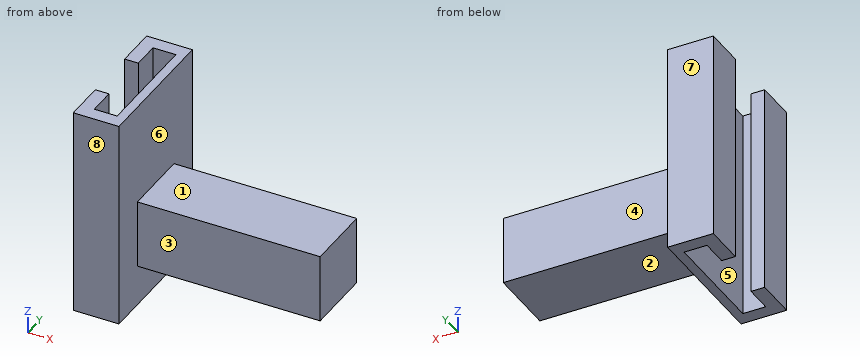
```python
from build123d import *

# Parameters (mm, degrees)
PAD_DEPTH    = 46
SKETCH002_W  = 14.95
SKETCH002_H  = 14.95
PAD001_DEPTH = 40


with BuildPart() as part:
    # Sketch → Pad (new body)
    with BuildSketch(Plane.XY):
        Polygon((-10, 15), (0, 15), (0, -15), (-10, -15), (-10, -6), (-7, -6), (-7, -12), (-2, -12), (-2, 12), (-7, 12), (-7, 6), (-10, 6), align=None)
    extrude(amount=PAD_DEPTH)

    # Sketch002 (on Face2 of Pad) → Pad001 (join)
    with BuildSketch(Plane.YZ):
        with Locations((0, 16.475)):
            Rectangle(SKETCH002_W, SKETCH002_H)
    extrude(amount=PAD001_DEPTH)


solid = part.part
```
Design review of the part built by this model. Coordinates are the model's own, in mm. Face numbers are marked on the shaded views. A direction names the side the tool comes from. Give positions to 0.01 mm unless a question says otherwise; leave off trailing zeros. Order: outer loops, then holes, each group sorted by start corner. A loop starts at its lowest first (then second) coordinate and runs counter-clockwise, first axis right, second up. Notation, with made-up numbers: (4.5, -26) - (57.5, -26) arc R29 ccw to (57.5, 10) - close; hole circle Ø7 at (87, 71). An arc over 180 degrees is marked (long way). Use a Markdown table: item, result. Add a question column.
(1) Add section B-B on x = -4.5. Give the boundary of the cut face in (y, z), then the cut area to 3 significant figures.
(2) Add section C-C on y = 5. Give the boundary of the cut face in (x, z), then the cut area to 3 significant figures.
(3) Machinability: for the marked faces 1, 2, 3 and 4, which of the approach directions +Z, -Z, +X, -X, +Y, -Y give a long, thin tool a straight path to every point of the face, cutting with its end or side? Answer none if there is none.
(4) Clearance check with flat-ended pins moving along their axes: P1, Ø8, axis at x = 9.5, z = 10.5, coming from the +Y side (3 decimals); P2, Ø8, axis at x = 29, z = 13, coming from the -Y side (3 decimals); P3, Ø7.5, axis at x = 18.5, y = 2.5, coming from the -Z side. State where each tip first meets the part, or that it passes through.
(5) Wall thickness on probe 1 along X at (y, z) = (-8, 23); probe 2 along X at (y, z) = (7, 10); probe 3 along Y at (x, z) = (-4, 5): over which ranges is each line inside the solid? List them lowest first. Write a range as [from, to].
(6) Add section A-A on y = -11.25. Give the boundary of the cut face in (x, z), then the cut area to 3 significant figures.
(7) Mouldability with a two-part tool opening along Y and no side actions: class the marked faces 5, 6, 7 and 8 as +Y half, -Y half, draft (parallel to the pull), parting line (faces both ways), or undercut.
(8) Add section D-D on z = 16. Give the boundary of the cut face in (x, y) (3 decimals), then the cut area to 3 significant figures.
Report:
| question | item | result |
|---|---|---|
| 1 | outline | (-15, 0) - (-12, 0) - (-12, 46) - (-15, 46) - close; (12, 0) - (15, 0) - (15, 46) - (12, 46) - close |
| 1 | area | 276 mm² |
| 2 | outline | (-2, 0) - (0, 0) - (0, 9) - (40, 9) - (40, 23.95) - (0, 23.95) - (0, 46) - (-2, 46) - close |
| 2 | area | 690 mm² |
| 3 | face 1 | +Z, +X, +Y, -Y |
| 3 | face 2 | -Z, +X, +Y, -Y |
| 3 | face 3 | +Z, -Z, +X, -Y |
| 3 | face 4 | +Z, -Z, +X, +Y |
| 4 | P1 | stops at y = 7.475 |
| 4 | P2 | stops at y = -7.475 |
| 4 | P3 | stops at z = 9 |
| 5 | probe 1 | x = [-10, -7], [-2, 0] |
| 5 | probe 2 | x = [-10, -7], [-2, 40] |
| 5 | probe 3 | y = [-15, -12], [12, 15] |
| 6 | outline | (-10, 0) - (-7, 0) - (-7, 46) - (-10, 46) - close; (-2, 0) - (0, 0) - (0, 46) - (-2, 46) - close |
| 6 | area | 230 mm² |
| 7 | face 5 | undercut |
| 7 | face 6 | draft |
| 7 | face 7 | +Y half |
| 7 | face 8 | -Y half |
| 8 | outline | (-10, -15) - (0, -15) - (0, -7.475) - (40, -7.475) - (40, 7.475) - (0, 7.475) - (0, 15) - (-10, 15) - (-10, 6) - (-7, 6) - (-7, 12) - (-2, 12) - (-2, -12) - (-7, -12) - (-7, -6) - (-10, -6) - close |
| 8 | area | 742 mm² |
